Source: CAD feature listing. Evaluate the final solid. Frame: model axes, mm. Face numbers are marked on the shaded views. Coordinates: 2 decimals unless noted, no trailing zeros. Write each loop counter-clockwise with the first axis right and the second up, starting at its lowest first coordinate (ties: lowest second). Pieces come first, ordered by that corner, then holes. Notation, with made-up numbers: (51, 70) - (108, 70) arc R28 ccw to (108, 109) - close; hole circle Ø7 at (-7, 7). An arc over 180 degrees is marked (long way). One line per item, written item: value.
Autodesk Inventor part; units mm, degrees
ref_plane "YZ Plane" through (0, 0, 0) normal (1, 0, 0) x (0, 1, 0)
ref_plane "XZ Plane" through (0, 0, 0) normal (0, 1, 0) x (-1, 0, 0)
ref_plane "XY Plane" through (0, 0, 0) normal (0, 0, 1) x (1, 0, 0)
sketch "Эскиз1" plane through (0, 0, 0) normal (1, 0, 0) x (0, 1, 0)
  line L0 (-17.5, 21) -> (-21, 17.5)
  line L1 (-21, 17.5) -> (-21, -17.5)
  line L2 (-21, -17.5) -> (-17.5, -21)
  line L3 (-17.5, -21) -> (17.5, -21)
  line L4 (17.5, -21) -> (21, -17.5)
  line L5 (21, -17.5) -> (21, 17.5)
  line L6 (21, 17.5) -> (17.5, 21)
  line L7 (17.5, 21) -> (-17.5, 21)
  line L8 (-21, 17.5) -> (-51, 17.5)
  line L9 (-51, 17.5) -> (-51, -17.5)
  line L10 (-51, -17.5) -> (-21, -17.5)
  line L11 (-21, -17.5) -> (-21, 17.5)
  line L12 (-51, 0) -> (-36, 0)
  line L13 (-36, 0) -> (-36, 10)
  line L14 (-36, 10) -> (-36, -10)
  circle A0 centre (-36, 10) radius 4
  circle A1 centre (-36, -10) radius 4
  line L15 (0, 17) -> (0, -17) construction
  line L16 (-2, 17) -> (-2, -17)
  line L17 (2, -17) -> (2, 17)
  arc A2 (2, 17) -> (-2, 17) centre (0, 17) ccw
  arc A3 (-2, -17) -> (2, -17) centre (0, -17) ccw
  point P0 (0, 0)
  point P1 (0, 0)
  point P2 (0, 0)
  dimension "d0" = 30
  dimension "d1" = 15
  dimension "d2" = 10
  dimension "d3" = 20
  dimension "d4" = 8
  dimension "d5" = 8
  dimension "d12" = 17
  dimension "d13" = 4
extrude "Выдавливание1" add sketch "Эскиз1" along normal blind 4
chamfer "Фаска1" distance 5 angle 45 2 edges at (2, -51, 17.5) (2, -51, -17.5)
properties part number "КВ33.044.002 - Держатель катка" material "Пластик АБС"
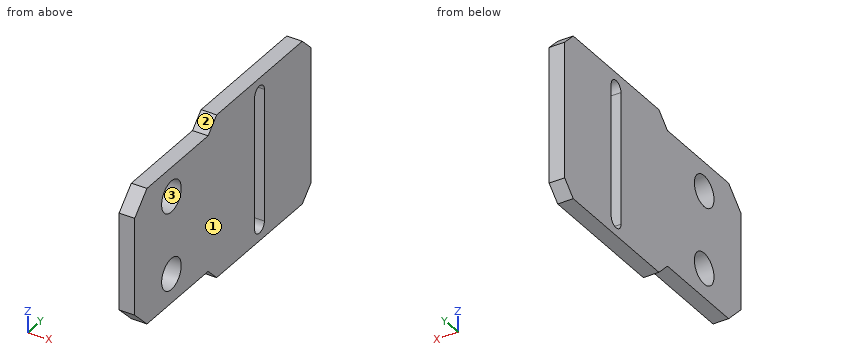
1) Contact query for flat-ended pins moving along their axis: P1, Ø1.2, axis at x = 2, y = -33, coming from the +Z side; P2, Ø10, axis at y = 6, z = 13.5, coming from the -X side. Output: stop coordinate, or through.
Values found:
P1: z = 17.5
P2: x = 0
2) Section query D-D on x = 1.55. Output: boundary loops of the cut face in (y, z), then the cut area to 3 significant figures.
Values found:
outline: (-51, -12.5) - (-46, -17.5) - (-21, -17.5) - (-17.5, -21) - (17.5, -21) - (21, -17.5) - (21, 17.5) - (17.5, 21) - (-17.5, 21) - (-21, 17.5) - (-46, 17.5) - (-51, 12.5) - close; hole circle Ø8 at (-36, -10); hole circle Ø8 at (-36, 10); hole (-2, -17) arc R2 ccw to (2, -17) - (2, 17) arc R2 ccw to (-2, 17) - close
area: 2,520 mm2
3) Section query B-B on z = -4. Output: boundary loops of the cut face in (x, y), then the cut area to 3 significant figures.
Values found:
outline: (0, -51) - (4, -51) - (4, -2) - (0, -2) - close; (0, 2) - (4, 2) - (4, 21) - (0, 21) - close
area: 272 mm2
4) Material intervals for line 1 (Y direction, x = 2.35, z = -10); line 2 (Z direction, x = 2.3, y = -36); line 3 (Y direction, x = 2.8, z = -0.5), sorted ascending.
Values found:
line 1: -51 to -40, -32 to -2, 2 to 21
line 2: -17.5 to -14, -6 to 6, 14 to 17.5
line 3: -51 to -2, 2 to 21
5) Draft query along Z for the marked faces 1, 2 and 3. Return one class per face: released by +Z, released by -Z, zero draft, split by the parting line, or undercut.
Values found:
face 1: zero draft
face 2: released by +Z
face 3: undercut
6) Section query A-A on y = 0. Output: boundary loops of the cut face in (x, z), then the cut area to 3 significant figures.
Values found:
outline: (0, -21) - (4, -21) - (4, -19) - (0, -19) - close; (0, 19) - (4, 19) - (4, 21) - (0, 21) - close
area: 16.0 mm2
7) Section query C-C on y = -36. Output: boundary loops of the cut face in (x, z), then the cut area to 3 significant figures.
Values found:
outline: (0, -17.5) - (4, -17.5) - (4, -14) - (0, -14) - close; (0, -6) - (4, -6) - (4, 6) - (0, 6) - close; (0, 14) - (4, 14) - (4, 17.5) - (0, 17.5) - close
area: 76.0 mm2
